from build123d import *

# Parameters (mm, degrees)
SKETCH003_W             = 15.88
SKETCH003_H             = 22.34
PAD001_DEPTH            = 7.7
POCKET002_DEPTH         = 5.7
POCKET003_DEPTH         = 2.52
SKETCH007_W             = 5.44
SKETCH007_H             = 2.67
POCKET004_DEPTH         = 5.7
POCKET005_DEPTH         = 7.701
POCKET006_DEPTH         = 2
POCKET007_DEPTH         = 1.1
FILLET_R                = 1
FILLET001_R             = 2
FILLET011_R             = 0.5
BODY001_PLACEMENT_ANGLE = 270


with BuildPart() as part:
    # Sketch003 (on XY_Plane013 of Origin026) → Pad001 (new body)
    with BuildSketch(Plane.XY):
        Rectangle(SKETCH003_W, SKETCH003_H)
    extrude(amount=PAD001_DEPTH)

    # Sketch004 (on XY_Plane013 of Origin026) → Pocket002 (cut)
    with BuildSketch(Plane.XY):
        with BuildLine():
            Line((-3.69, 8.67), (3.69, 8.67))
            ThreePointArc((5.44, 6.92), (4.927437, 8.157437), (3.69, 8.67))
            Line((5.44, 6.92), (5.44, -6.92))
            ThreePointArc((3.69, -8.67), (4.927437, -8.157437), (5.44, -6.92))
            Line((3.69, -8.67), (-3.69, -8.67))
            ThreePointArc((-5.44, -6.92), (-4.927437, -8.157437), (-3.69, -8.67))
            Line((-5.44, -6.92), (-5.44, 6.92))
            ThreePointArc((-3.69, 8.67), (-4.927437, 8.157437), (-5.44, 6.92))
        make_face()
    extrude(amount=POCKET002_DEPTH, mode=Mode.SUBTRACT)

    # Sketch006 (on XY_Plane013 of Origin026) → Pocket003 (cut)
    with BuildSketch(Plane.XY):
        with BuildLine():
            Line((5.99, 6.92), (5.99, -6.92))
            ThreePointArc((3.69, -9.22), (5.316346, -8.546346), (5.99, -6.92))
            Line((3.69, -9.22), (-3.69, -9.22))
            ThreePointArc((-5.99, -6.92), (-5.316346, -8.546346), (-3.69, -9.22))
            Line((-5.99, -6.92), (-5.99, 6.92))
            ThreePointArc((-3.69, 9.22), (-5.316346, 8.546346), (-5.99, 6.92))
            Line((-3.69, 9.22), (-3.47, 9.22))
            ThreePointArc((-3.47, 9.22), (-2.93967, 9.43967), (-2.72, 9.97))
            Line((-2.72, 11.17), (-2.72, 9.97))
            Line((2.72, 11.17), (-2.72, 11.17))
            Line((2.72, 11.17), (2.72, 9.97))
            ThreePointArc((2.72, 9.97), (2.93967, 9.43967), (3.47, 9.22))
            Line((3.69, 9.22), (3.47, 9.22))
            ThreePointArc((5.99, 6.92), (5.316346, 8.546346), (3.69, 9.22))
        make_face()
    extrude(amount=POCKET003_DEPTH, mode=Mode.SUBTRACT)

    # Sketch007 (on XY_Plane013 of Origin026) → Pocket004 (cut)
    with BuildSketch(Plane.XY):
        with Locations((0, 9.835)):
            Rectangle(SKETCH007_W, SKETCH007_H)
    extrude(amount=POCKET004_DEPTH, mode=Mode.SUBTRACT)

    # Sketch008 (on XY_Plane013 of Origin026) → Pocket005 (cut, through all)
    with BuildSketch(Plane.XY):
        with BuildLine():
            Line((2.72, 11.17), (2.72, 9.97))
            ThreePointArc((1.97, 9.22), (2.50033, 9.43967), (2.72, 9.97))
            Line((1.97, 9.22), (-1.97, 9.22))
            ThreePointArc((-2.72, 9.97), (-2.50033, 9.43967), (-1.97, 9.22))
            Line((-2.72, 11.17), (-2.72, 9.97))
            Line((2.72, 11.17), (-2.72, 11.17))
        make_face()
    extrude(amount=POCKET005_DEPTH, mode=Mode.SUBTRACT)

    # Sketch009 (on XY_Plane013 of Origin026) → Pocket006 (cut)
    with BuildSketch(Plane.XY.offset(7.7)):
        with BuildLine():
            Line((-0.77, -0.58), (-0.77, -7.7))
            ThreePointArc((-1.52, -8.45), (-0.98967, -8.23033), (-0.77, -7.7))
            Line((-3.56, -8.45), (-1.52, -8.45))
            ThreePointArc((-4.31, -7.7), (-4.09033, -8.23033), (-3.56, -8.45))
            Line((-4.31, -7.7), (-4.31, -0.58))
            ThreePointArc((-3.56, 0.17), (-4.09033, -0.04967), (-4.31, -0.58))
            Line((-3.56, 0.17), (-1.52, 0.17))
            ThreePointArc((-0.77, -0.58), (-0.98967, -0.04967), (-1.52, 0.17))
        make_face()
        with BuildLine():
            Line((0.77, -0.58), (0.77, -7.7))
            ThreePointArc((0.77, -7.7), (0.98967, -8.23033), (1.52, -8.45))
            Line((1.52, -8.45), (3.56, -8.45))
            ThreePointArc((3.56, -8.45), (4.09033, -8.23033), (4.31, -7.7))
            Line((4.31, -7.7), (4.31, -0.58))
            ThreePointArc((4.31, -0.58), (4.09033, -0.04967), (3.56, 0.17))
            Line((1.52, 0.17), (3.56, 0.17))
            ThreePointArc((1.52, 0.17), (0.98967, -0.04967), (0.77, -0.58))
        make_face()
    extrude(amount=-POCKET006_DEPTH, mode=Mode.SUBTRACT)

    # Sketch010 (on XY_Plane013 of Origin026) → Pocket007 (cut)
    with BuildSketch(Plane.XY):
        with BuildLine():
            Line((5.23, 13.43), (10.23, 13.43))
            Line((10.23, 13.43), (10.23, 8.43))
            Line((6.63, 8.43), (10.23, 8.43))
            ThreePointArc((5.23, 9.83), (4.240051, 7.440051), (6.63, 8.43))
            Line((5.23, 9.83), (5.23, 13.43))
        make_face()
        with BuildLine():
            Line((-5.23, 13.43), (-10.23, 13.43))
            Line((-10.23, 13.43), (-10.23, 8.43))
            Line((-10.23, 8.43), (-6.63, 8.43))
            ThreePointArc((-6.63, 8.43), (-4.240051, 7.440051), (-5.23, 9.83))
            Line((-5.23, 13.43), (-5.23, 9.83))
        make_face()
        with BuildLine():
            Line((5.23, -13.43), (10.23, -13.43))
            Line((10.23, -13.43), (10.23, -8.43))
            Line((6.63, -8.43), (10.23, -8.43))
            ThreePointArc((6.63, -8.43), (4.240051, -7.440051), (5.23, -9.83))
            Line((5.23, -13.43), (5.23, -9.83))
        make_face()
        with BuildLine():
            Line((-10.23, -13.43), (-5.23, -13.43))
            Line((-5.23, -13.43), (-5.23, -9.83))
            ThreePointArc((-5.23, -9.83), (-4.240051, -7.440051), (-6.63, -8.43))
            Line((-10.23, -8.43), (-6.63, -8.43))
            Line((-10.23, -13.43), (-10.23, -8.43))
        make_face()
    extrude(amount=POCKET007_DEPTH, mode=Mode.SUBTRACT)

    # Fillet
    fillet_edges = [part.edges().sort_by_distance(p)[0] for p in [
        (2.72, 11.17, 3.85),
        (-2.72, 11.17, 3.85),
    ]]
    fillet(fillet_edges, radius=FILLET_R)

    # Fillet001
    fillet001_edges = [part.edges().sort_by_distance(p)[0] for p in [
        (7.94, 11.17, 4.4),
        (-7.94, 11.17, 4.4),
        (-7.94, -11.17, 4.4),
        (7.94, -11.17, 4.4),
    ]]
    fillet(fillet001_edges, radius=FILLET001_R)

    # Fillet011
    fillet011_edges = [part.edges().sort_by_distance(p)[0] for p in [
        (2.72, 8.67, 4.11),
        (-2.72, 8.67, 4.11),
    ]]
    fillet(fillet011_edges, radius=FILLET011_R)


with BuildPart() as part_1:
    # Body001 placement: moved
    add(part.part.moved(Location((0, 9.33, 43.08))).rotate(Axis((0, 9.33, 43.08), (1, 0, 0)), BODY001_PLACEMENT_ANGLE))


solid = part_1.part
Could you check a few things on this model? Use its own coordinates, in mm. A direction names the side the tool comes from. Coordinates: 2 decimals unless noted, no trailing zeros. Order: outer loops, then holes, each group sorted by start corner. A loop starts at its lowest first (then second) coordinate and runs counter-clockwise, first axis right, second up. Notation, with made-up numbers: (57, 51) -> (87, 51) arc R35 ccw to (87, 87) -> close; hole circle Ø5 at (46, 51.25). An arc over 180 degrees is marked (long way). One line per item, written item: value. Start each with the question number.
1) Imagine slicing it at A-A on z = 46.5. List the corners of the cut face in (x, y) for me, plus the area to 3 significant figures.
2) Which directions (+Z, -Z, +X, -X, +Y, -Y) give clear straight access to the entire face, cutting with the end or side of a thin tool? Please do faces 1 (the flat face through (3, 16, 51.53)), 2 (the cylindrical face through (-6.45, 9.87, 50.82)), 3 (the cylindrical face through (6.45, 9.87, 35.34)), 4 (the flat face through (5.23, 10, 54)), 5 (the flat face through (6, 10.43, 33)).
3) I'm going to push flat-ended pins straight in: pin 1 (6 mm diameter, centred on x = -1.5, z = 39, fed in from -Y); pin 2 (1 mm diameter, centred on x = 1, y = 16.5, fed in from -Z); pin 3 (2 mm diameter, centred on x = -1.5, y = 10.5, fed in from -Z). Where does each tip first touch, or does it pass through?
4) Imagine slicing it at D-D on y = 11.5. List the corners of the cut face in (x, z) for me, plus the area to 3 significant figures.
5) If I drill on L1, parallel to X at y = 14.75, z = 45; L2, parallel to X at y = 11.5, z = 36.75; L3, parallel to Z at x = 4.25, y = 11.5, over which ranges is the centre line in solid material (lowest first)? Write a range as [from, to].
6) We'd pull the mould along X, two halves only. Please class faces 6 (the flat face through (7, 9.33, 43)), 7 (the cylindrical face through (6.46, 9.87, 50.84)), 8 (the cylindrical face through (7.37, 13.78, 32.51)): +X half, -X half, draft (parallel to the pull), parting line (faces both ways), or undercut.
7) Imagine slicing it at C-C on z = 41. List the corners of the cut face in (x, y) for me, plus the area to 3 significant figures.
8) Imagine slicing it at B-B on x = 1. List the corners of the cut face in (y, z) for me, plus the area to 3 significant figures.
Answer list:
1. outline: (-7.94, 9.33) -> (-5.99, 9.33) -> (-5.99, 11.85) -> (-5.44, 11.85) -> (-5.44, 15.03) -> (-4.31, 15.03) -> (-4.31, 17.03) -> (-7.94, 17.03) -> close; (-0.77, 15.03) -> (0.77, 15.03) -> (0.77, 17.03) -> (-0.77, 17.03) -> close; (4.31, 15.03) -> (5.44, 15.03) -> (5.44, 11.85) -> (5.99, 11.85) -> (5.99, 9.33) -> (7.94, 9.33) -> (7.94, 17.03) -> (4.31, 17.03) -> close
1. area: 43.3 mm2
2. face 1: +Y, -Y
2. face 2: +Z, -Y
2. face 3: -Z, -Y
2. face 4: +Z, -Z, +X, -Y
2. face 5: -Y
3. pin 1: stops at y = 15.03
3. pin 2: stops at z = 33.86
3. pin 3: stops at z = 52.3
4. outline: (-7.94, 33.91) arc R2 ccw to (-5.94, 31.91) -> (-3.72, 31.91) arc R1 ccw to (-2.72, 32.91) -> (-2.72, 33.11) arc R0.75 ccw to (-3.47, 33.86) -> (-3.69, 33.86) arc R2.3 cw to (-5.99, 36.16) -> (-5.99, 50) arc R2.3 cw to (-3.69, 52.3) -> (3.69, 52.3) arc R2.3 cw to (5.99, 50) -> (5.99, 36.16) arc R2.3 cw to (3.69, 33.86) -> (3.47, 33.86) arc R0.75 ccw to (2.72, 33.11) -> (2.72, 32.91) arc R1 ccw to (3.72, 31.91) -> (5.94, 31.91) arc R2 ccw to (7.94, 33.91) -> (7.94, 52.25) arc R2 ccw to (5.94, 54.25) -> (-5.94, 54.25) arc R2 ccw to (-7.94, 52.25) -> close
4. area: 124 mm2
5. L1: x = [-7.94, -5.44], [5.44, 7.94]
5. L2: x = [-7.94, -5.99], [5.99, 7.94]
5. L3: z = [31.91, 33.93], [52.23, 54.25]
6. face 6: draft
6. face 7: undercut
6. face 8: +X half
7. outline: (-7.94, 9.33) -> (-5.99, 9.33) -> (-5.99, 11.85) -> (-5.44, 11.85) -> (-5.44, 15.03) -> (5.44, 15.03) -> (5.44, 11.85) -> (5.99, 11.85) -> (5.99, 9.33) -> (7.94, 9.33) -> (7.94, 17.03) -> (-7.94, 17.03) -> close
7. area: 57.5 mm2
8. outline: (9.33, 52.3) -> (11.85, 52.3) -> (11.85, 51.75) -> (15.03, 51.75) -> (15.03, 51.32) -> (17.03, 51.32) -> (17.03, 54.25) -> (9.33, 54.25) -> close; (15.03, 33.86) -> (17.03, 33.86) -> (17.03, 43.12) -> (15.03, 43.12) -> close
8. area: 37.2 mm2
